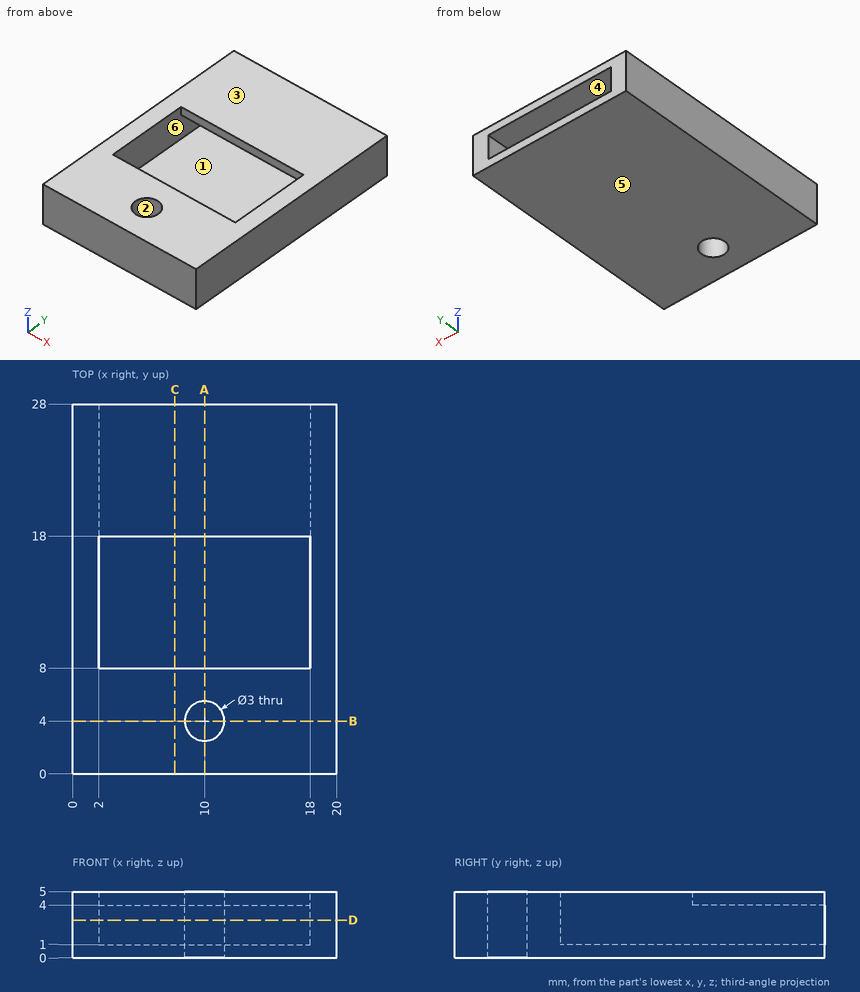
Job drawing, mm, ordinate dimensions from the low corner. One solid piece. A direction names the side the tool comes from. Give positions to 0.01 mm unless a question says otherwise; leave off trailing zeros. Write each loop counter-clockwise with the first axis right and the second up, starting at its lowest first coordinate (ties: lowest second). Pieces come first, ordered by that corner, then holes. Notation, with made-up numbers: (78.25, 53.5) - (87.25, 53.5) arc R25 ccw to (87.25, 66.5) - close; hole circle Ø8 at (-9.75, -38.75). An arc over 180 degrees is marked (long way). Use one line per item in the form item = value. Start each with the question number.
1. Probe line 1 (X direction, y = 26, z = 2.3); line 2 (Y direction, x = 10, z = 3.7); line 3 (Y direction, x = 5.5, z = 1.1). List the from-to ranges inside material, lowest first. Write a range as [from, to].
2. Drop a flat-ended pin along its axis: pin 1 Ø5 at (x, y) = (10.5, 12) entering from +Z. Give the stop position or say it passes through.
3. Band-saw the part on C-C on x = 7.75. Write the cut outline in (y, z).
4. Two-plate mould, pull along Z, no slides. Class the marked faces 3, 4, 5 and 6: released by +Z, released by -Z, zero draft, split by the parting line, or undercut.
5. Band-saw the part on D-D on z = 2.85. Write the cut outline in (x, y).
6. Band-saw the part on B-B on y = 4. Write the cut outline in (x, z), plus the area to 3 significant figures.
7. Band-saw the part on A-A on x = 10. Write the cut outline in (y, z).
8. 3-axis set-ups, long thin cutter, end or side, ignore diameter. For the marked faces 1 and 2: which of +Z, -Z, +X, -X, +Y, -Y reach the whole face in a straight line?
Conclusion:
q1.line_1 = [0, 2], [18, 20]
q1.line_2 = [0, 2.5], [5.5, 8]
q1.line_3 = [0, 8]
q2.pin_1 = 1
q3.outline = (0, 0) - (28, 0) - (28, 1) - (8, 1) - (8, 5) - (0, 5) - close; (18, 4) - (28, 4) - (28, 5) - (18, 5) - close
q4.face_3 = released by +Z
q4.face_4 = undercut
q4.face_5 = released by -Z
q4.face_6 = undercut
q5.outline = (0, 0) - (20, 0) - (20, 28) - (18, 28) - (18, 8) - (2, 8) - (2, 28) - (0, 28) - close; hole circle Ø3 at (10, 4)
q6.outline = (0, 0) - (8.5, 0) - (8.5, 5) - (0, 5) - close; (11.5, 0) - (20, 0) - (20, 5) - (11.5, 5) - close
q6.area = 85.0 mm²
q7.outline = (0, 0) - (2.5, 0) - (2.5, 5) - (0, 5) - close; (5.5, 0) - (28, 0) - (28, 1) - (8, 1) - (8, 5) - (5.5, 5) - close; (18, 4) - (28, 4) - (28, 5) - (18, 5) - close
q8.face_1 = +Y
q8.face_2 = +Z, -Z
